from build123d import *

# Parameters (mm, degrees)
SKETCH007_R     = 2.45
PAD007_DEPTH    = 7
POCKET_START    = -2
SKETCH008_R     = 1.6
POCKET_DEPTH    = 6
SKETCH_R        = 4
PAD_DEPTH       = 10
POCKET001_START = -16
SKETCH010_R     = 2.5
POCKET001_DEPTH = 9
PAD008_DEPTH    = 7


with BuildPart() as part:
    # Sketch007 → Pad007 (new body)
    with BuildSketch(Plane.XY):
        with Locations((4, 4)):
            Circle(SKETCH007_R)
    extrude(amount=-PAD007_DEPTH)

    # Sketch008 → Pocket (cut)
    with BuildSketch(Plane.XY.offset(POCKET_START)):
        with Locations((4, 4)):
            Circle(SKETCH008_R)
    extrude(amount=-POCKET_DEPTH, mode=Mode.SUBTRACT)

    # Sketch → Pad (join)
    with BuildSketch(Plane.XY):
        with Locations((4, 4)):
            Circle(SKETCH_R)
    extrude(amount=PAD_DEPTH)

    # Sketch010 → Pocket001 (cut)
    with BuildSketch(Plane(origin=(0, 0, -15), x_dir=(1, 0, 0), z_dir=(0, 0, -1)).offset(POCKET001_START)):
        with Locations((4, -4)):
            Circle(SKETCH010_R)
    extrude(amount=-POCKET001_DEPTH, mode=Mode.SUBTRACT)

    # Sketch009 → Pad008 (join)
    with BuildSketch(Plane.XY):
        with BuildLine():
            ThreePointArc((5.541903, 5.967876), (4, 6.5), (2.458097, 5.967876))
            Line((2.458097, 5.967876), (5.541903, 5.967876))
        make_face()
        with BuildLine():
            ThreePointArc((2.456381, 2.03347), (4, 1.5), (5.543619, 2.03347))
            Line((2.456381, 2.03347), (5.543619, 2.03347))
        make_face()
    extrude(amount=PAD008_DEPTH)


solid = part.part
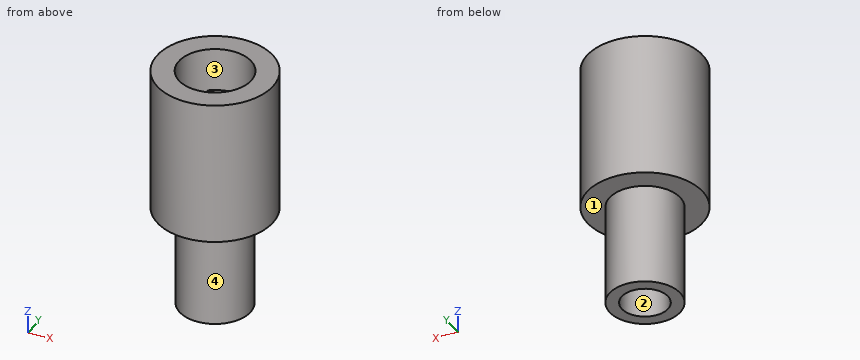
Could you check a few things on this model? Use its own coordinates, in mm. Face numbers are marked on the shaded views. Give positions to 0.01 mm unless a question says otherwise; leave off trailing zeros. Order: outer loops, then holes, each group sorted by start corner. A loop starts at its lowest first (then second) coordinate and runs counter-clockwise, first axis right, second up. Notation, with made-up numbers: (-24.5, 60.25) -> (-0.5, 60.25) arc R20 ccw to (-0.5, 69.25) -> close; hole circle Ø3 at (6, 17.5). An arc over 180 degrees is marked (long way). Return JSON: item names as keys, results as strings.
1. Imagine slicing it at A-A on y = 4. List the corners of the cut face in (x, z) for me, then the cut area to 3 significant figures.
Answer list:
{"outline": "(0, 0) -> (1.55, 0) -> (1.55, -7) -> (2.4, -7) -> (2.4, -2) -> (5.6, -2) -> (5.6, -7) -> (6.45, -7) -> (6.45, 0) -> (8, 0) -> (8, 10) -> (6.5, 10) -> (6.5, 1) -> (1.5, 1) -> (1.5, 10) -> (0, 10) -> close", "area": "53.3 mm2"}
2. I need wall thicknesses on line 1 (Y direction, x = 4, z = 6.25); line 2 (Y direction, x = 4, z = 7.25); line 3 (Z direction, x = 1.5, y = 1). Which ranges of each line are inside material? Lowest first, please. Write a range as from..to.
Answer list:
{"line 1": "y = 0..2.03, 5.97..8", "line 2": "y = 0..1.5, 6.5..8", "line 3": "z = 0..10"}
3. Imagine slicing it at C-C on z = 4.75. List the corners of the cut face in (x, y) for me, then the cut area to 3 significant figures.
Answer list:
{"outline": "circle Ø8 at (4, 4); hole (2.46, 2.03) -> (5.54, 2.03) arc R2.5 ccw to (5.54, 5.97) -> (2.46, 5.97) arc R2.5 ccw to start", "area": "32.9 mm2"}
4. Imagine slicing it at D-D on z = 0.5. List the corners of the cut face in (x, y) for me.
Answer list:
{"outline": "circle Ø8 at (4, 4)"}
5. Thinking about a two-plate mould opening in X: for the marked faces 1, 2, 3 and 4, which applies, pulls with the +X half, pulls with the -X half, needs draft (parallel to the pull), parting line crosses it, or undercut?
Answer list:
{"face 1": "needs draft", "face 2": "undercut", "face 3": "undercut", "face 4": "parting line crosses it"}
6. Imagine slicing it at B-B on x = 4. List the corners of the cut face in (y, z) for me, then the cut area to 3 significant figures.
Answer list:
{"outline": "(0, 0) -> (1.55, 0) -> (1.55, -7) -> (2.4, -7) -> (2.4, -2) -> (5.6, -2) -> (5.6, -7) -> (6.45, -7) -> (6.45, 0) -> (8, 0) -> (8, 10) -> (6.5, 10) -> (6.5, 7) -> (5.97, 7) -> (5.97, 1) -> (2.03, 1) -> (2.03, 7) -> (1.5, 7) -> (1.5, 10) -> (0, 10) -> close", "area": "59.7 mm2"}
7. For pin 1 Ø1.9 at (x, y) = (4, 4) entering from -Z; pin 2 Ø1.5 at (x, z) = (7, -1.5) entering from -Y; pin 3 Ø2 at (x, y) = (3, 4) entering from +Z, each with a flat end and sliding along its axis, tell me the tip position at first contact or that it passes through.
Answer list:
{"pin 1": "stops at z = -2", "pin 2": "stops at y = 3.03", "pin 3": "stops at z = 1"}
